```python
from build123d import *

# Parameters (mm, degrees)
SKETCH1_W           = 32.9
SKETCH1_H           = 22.4
BOSS_EXTRUDE1_DEPTH = 5
SKETCH2_R           = 1.2
SKETCH2_W           = 22.9
SKETCH2_H           = 12.4
CUT_EXTRUDE2_DEPTH  = 5
SKETCH3_W           = 22.996888994
SKETCH3_H           = 5
BOSS_EXTRUDE2_DEPTH = 12.3
SKETCH4_R           = 1.2
CUT_EXTRUDE3_DEPTH  = 5
SKETCH6_W           = 5
SKETCH6_H           = 5
SKETCH6_W_2         = 4.903111006
BOSS_EXTRUDE3_DEPTH = 12.3
SKETCH8_W           = 17.3
SKETCH8_H           = 4.998204887
BOSS_EXTRUDE4_DEPTH = 3.1
SKETCH9_W           = 17.3
SKETCH9_H           = 5
BOSS_EXTRUDE5_DEPTH = 3.1
SKETCH18_W          = 5
SKETCH18_H          = 12.4
BOSS_EXTRUDE7_DEPTH = 30
SKETCH19_R          = 4.5
CUT_EXTRUDE6_DEPTH  = 30
SKETCH20_R          = 4.5
CUT_EXTRUDE7_DEPTH  = 30
SKETCH10_W          = 5
SKETCH10_H          = 12.4
BOSS_EXTRUDE6_DEPTH = 30
SKETCH21_R          = 4.5
CUT_EXTRUDE8_DEPTH  = 10
SKETCH22_R          = 4.5
CUT_EXTRUDE9_DEPTH  = 10
CUT_EXTRUDE10_DEPTH = 3


with BuildPart() as part:
    # Sketch1 → Boss-Extrude1 (new body)
    with BuildSketch(Plane.XY):
        Rectangle(SKETCH1_W, SKETCH1_H)
    extrude(amount=BOSS_EXTRUDE1_DEPTH)

    # Sketch2 → Cut-Extrude2 (cut)
    with BuildSketch(Plane.XY.offset(5)):
        with Locations((13.8, 0)):
            Circle(SKETCH2_R)
        with Locations((-13.8, 0)):
            Circle(SKETCH2_R)
        Rectangle(SKETCH2_W, SKETCH2_H)
    extrude(amount=-CUT_EXTRUDE2_DEPTH, mode=Mode.SUBTRACT)

    # Sketch3 → Boss-Extrude2 (add)
    with BuildSketch(Plane.XY.offset(5)):
        with Locations((0.048444497, 8.7)):
            Rectangle(SKETCH3_W, SKETCH3_H)
        with Locations((0.048444497, -8.7)):
            Rectangle(SKETCH3_W, SKETCH3_H)
    extrude(amount=BOSS_EXTRUDE2_DEPTH)

    # Sketch4 → Cut-Extrude3 (cut)
    with BuildSketch(Plane.XY.offset(17.3)):
        with Locations((0.048444497, 8.7)):
            Circle(SKETCH4_R)
        with Locations((0.048444497, -8.7)):
            Circle(SKETCH4_R)
    extrude(amount=-CUT_EXTRUDE3_DEPTH, mode=Mode.SUBTRACT)

    # Sketch6 → Boss-Extrude3 (add)
    with BuildSketch(Plane.XY.offset(5)):
        with Locations((-13.95, -8.7)):
            Rectangle(SKETCH6_W, SKETCH6_H)
        with Locations((13.998444497, -8.7)):
            Rectangle(SKETCH6_W_2, SKETCH6_H)
    extrude(amount=BOSS_EXTRUDE3_DEPTH)

    # Sketch8 → Boss-Extrude4 (add)
    with BuildSketch(Plane(origin=(16.45, 0, 0), x_dir=(0, 0, -1), z_dir=(1, 0, 0))):
        with Locations((-8.65, -8.700897557)):
            Rectangle(SKETCH8_W, SKETCH8_H)
    extrude(amount=BOSS_EXTRUDE4_DEPTH)

    # Sketch9 → Boss-Extrude5 (add)
    with BuildSketch(Plane.ZY.offset(16.45)):
        with Locations((8.65, -8.7)):
            Rectangle(SKETCH9_W, SKETCH9_H)
    extrude(amount=BOSS_EXTRUDE5_DEPTH)

    # Sketch18 → Boss-Extrude7 (add)
    with BuildSketch(Plane.XZ.offset(11.2)):
        with Locations((-17.05, 8.65)):
            Rectangle(SKETCH18_W, SKETCH18_H)
        with Locations((17.05, 8.65)):
            Rectangle(SKETCH18_W, SKETCH18_H)
    extrude(amount=BOSS_EXTRUDE7_DEPTH)

    # Sketch19 → Cut-Extrude6 (cut)
    with BuildSketch(Plane.ZY.offset(19.55)):
        with Locations((8.65, -34.8)):
            Circle(SKETCH19_R)
    extrude(amount=-CUT_EXTRUDE6_DEPTH, mode=Mode.SUBTRACT)

    # Sketch20 → Cut-Extrude7 (cut)
    with BuildSketch(Plane(origin=(19.55, 0, 0), x_dir=(0, 0, -1), z_dir=(1, 0, 0))):
        with Locations((-8.65, -34.8)):
            Circle(SKETCH20_R)
    extrude(amount=-CUT_EXTRUDE7_DEPTH, mode=Mode.SUBTRACT)

    # Sketch10 → Boss-Extrude6 (add)
    with BuildSketch(Plane.XZ.offset(11.2)):
        with Locations((17.05, 8.65)):
            Rectangle(SKETCH10_W, SKETCH10_H)
        with Locations((-17.05, 8.65)):
            Rectangle(SKETCH10_W, SKETCH10_H)
    extrude(amount=BOSS_EXTRUDE6_DEPTH)

    # Sketch21 → Cut-Extrude8 (cut)
    with BuildSketch(Plane(origin=(19.55, 0, 0), x_dir=(0, 0, -1), z_dir=(1, 0, 0))):
        with Locations((-8.65, -34.8)):
            Circle(SKETCH21_R)
    extrude(amount=-CUT_EXTRUDE8_DEPTH, mode=Mode.SUBTRACT)

    # Sketch22 → Cut-Extrude9 (cut)
    with BuildSketch(Plane(origin=(-14.55, 0, 0), x_dir=(0, 0, -1), z_dir=(1, 0, 0))):
        with Locations((-8.65, -34.8)):
            Circle(SKETCH22_R)
    extrude(amount=-CUT_EXTRUDE9_DEPTH, mode=Mode.SUBTRACT)

    # Sketch23 → Cut-Extrude10 (cut)
    with BuildSketch(Plane.ZY.offset(19.55)):
        with BuildLine():
            Line((5.65, -22.3), (4.674239456, -32.692079676))
            ThreePointArc((4.674239456, -32.692079676), (8.65, -30.3), (12.625760544, -32.692079676))
            Line((12.625760544, -32.692079676), (11.65, -22.3))
            ThreePointArc((11.65, -22.3), (8.65, -19.3), (5.65, -22.3))
        make_face()
    extrude(amount=-CUT_EXTRUDE10_DEPTH, mode=Mode.SUBTRACT)


solid = part.part
```
The model under review builds one solid part; all positions refer to its coordinate system, in mm. A direction names the side the tool comes from. Give positions to 0.01 mm unless a question says otherwise; leave off trailing zeros. Loops run counter-clockwise (first coordinate to the right, second up) from the corner with the lowest first, then second, coordinate; pieces in that order, holes last. Notation, with made-up numbers: (17, 23.5) - (33, 23.5) arc R30 ccw to (33, 47.5) - close; hole circle Ø3 at (70, 57). An arc over 180 degrees is marked (long way). Answer as a JSON object with one key per item and string values.
Q1. Add section B-B on y = 0. State the section outline as (x, z) points.
Worked out:
{"outline": "(-16.45, 0) - (-15, 0) - (-15, 5) - (-16.45, 5) - close; (-12.6, 0) - (-11.45, 0) - (-11.45, 5) - (-12.6, 5) - close; (11.45, 0) - (12.6, 0) - (12.6, 5) - (11.45, 5) - close; (15, 0) - (16.45, 0) - (16.45, 5) - (15, 5) - close"}
Q2. Add section A-A on z = 13.75. Count the separate pieces of the cut face and the enclosed holes in it, plus the area to 3 significant figures.
Worked out:
{"separate pieces": "2", "enclosed holes": "2", "area": "601 mm^2"}
Q3. To check wall thickness, follow line 1 along Y through (x, z) = (-8, 5.75); line 2 along X through (y, z) = (-25, 8.25); line 3 along X through (y, z) = (-13, 4.25). State the ranges of each line that lie inside material, in increasing order.
Worked out:
{"line 1": "y = -11.2 to -6.2, 6.2 to 11.2", "line 2": "x = -16.55 to -14.55, 14.55 to 19.55", "line 3": "x = -19.55 to -14.55, 14.55 to 19.55"}
Q4. Add section D-D on z = 3.5. State the section outline as (x, y) points.
Worked out:
{"outline": "(-19.55, -41.2) - (-14.55, -41.2) - (-14.55, -11.2) - (14.55, -11.2) - (14.55, -41.2) - (19.55, -41.2) - (19.55, -6.2) - (16.45, -6.2) - (16.45, 11.2) - (-16.45, 11.2) - (-16.45, -6.2) - (-19.55, -6.2) - close; hole circle Ø2.4 at (-13.8, 0); hole (-11.45, -6.2) - (11.45, -6.2) - (11.45, 6.2) - (-11.45, 6.2) - close; hole circle Ø2.4 at (13.8, 0)"}
Q5. For faces 1 (the cylindrical face through (-18.1, -19.3, 8.7)), 2 (the flat face through (0, -9, 12.3)), 3 (the flat face through (-11.45, 0, 3)), 4 (the flat face through (-17, -26, 2.45)), 5 (the flat face through (-17, -26, 14.85)), list the 3-axis set-ups (+Z, -Z, +X, -X, +Y, -Y) from which the entire face can be reached by the end or side of a thin tool; tool diameter is ignored.
Worked out:
{"face 1": "-X", "face 2": "+Z", "face 3": "+Z, -Z", "face 4": "-Z, +X, -X, -Y", "face 5": "+Z, +X, -X, -Y"}
Q6. Add section C-C on x = 13.8. State the section outline as (y, z) points.
Worked out:
{"outline": "(-11.2, 0) - (-1.2, 0) - (-1.2, 5) - (-6.2, 5) - (-6.2, 17.3) - (-11.2, 17.3) - close; (1.2, 0) - (11.2, 0) - (11.2, 5) - (1.2, 5) - close"}
Q7. Insertion check: pin 1 (2.5 mm diameter, centred on x = -18, y = -26, fed in from +Z); pin 2 (4 mm diameter, centred on x = -2, z = 14, fed in from -Y); pin 3 (4 mm diameter, centred on x = 17.5, y = -22.5, fed in from -Z); pin 4 (5 mm diameter, centred on y = -33.5, z = 9.5, fed in from +X). Each pin has a flat end and moves straight along its axis. Give the tip position at first contact, or say it passes through.
Worked out:
{"pin 1": "stops at z = 14.85", "pin 2": "stops at y = -11.2", "pin 3": "stops at z = 2.45", "pin 4": "passes through"}
Q8. Mouldability with a two-part tool opening along Y and no side actions: class faces 6 (the flat face through (11.547, 9, 11)), 7 (the flat face through (-16.55, -26, 9)) as +Y half, -Y half, draft (parallel to the pull), parting line (faces both ways), or undercut.
Worked out:
{"face 6": "draft", "face 7": "undercut"}
